Answer from the drawing. Dimensions are ordinates in mm from the lowest x, y and z of the part. Coordinates: 2 decimals unless noted, no trailing zeros. Order: outer loops, then holes, each group sorted by start corner. A loop starts at its lowest first (then second) coordinate and runs counter-clockwise, first axis right, second up. Notation, with made-up numbers: (62, 61) -> (69, 61) arc R28 ccw to (69, 100) -> close; hole circle Ø4 at (39.5, 75). An arc over 180 degrees is marked (long way). Answer in a Markdown table with one row per item.
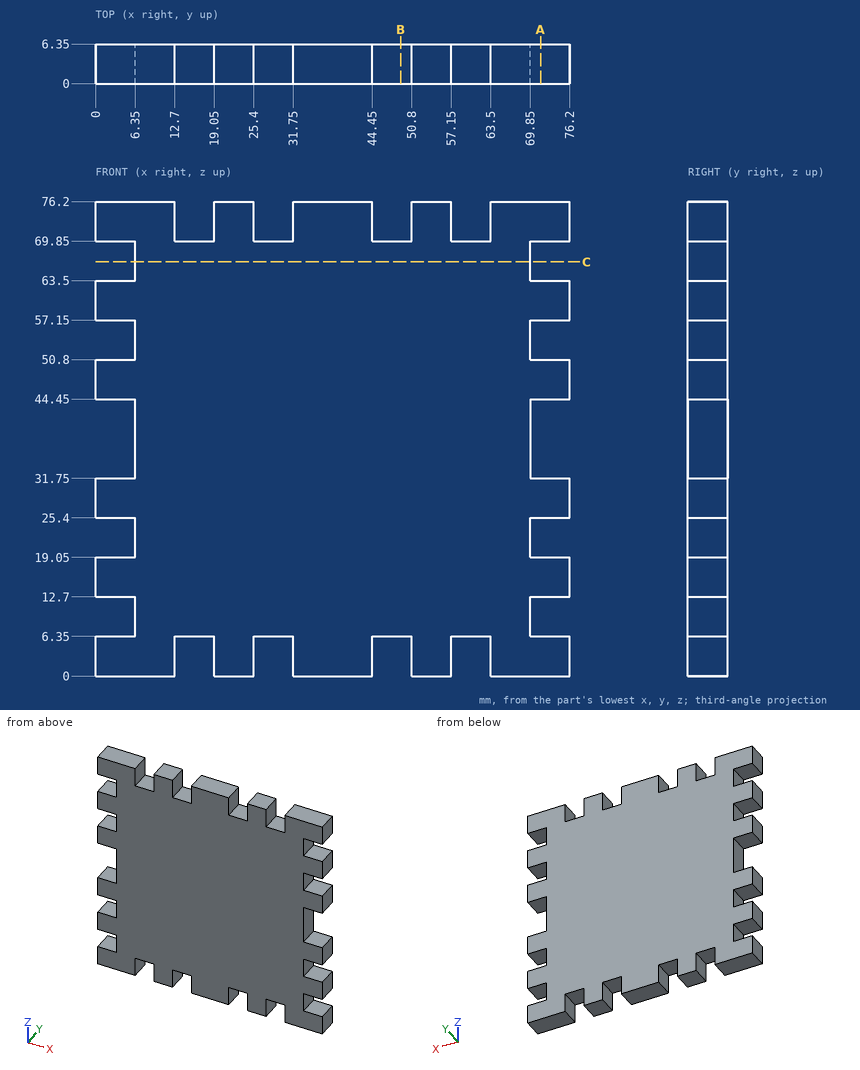
Q1. Consider line 1 (Z direction, x = 71.5, y = 5.25); line 2 (Z direction, x = 18, y = 4). Determine where each line is inside the solid, lowest interval first.
Outcome:
| item | result |
|---|---|
| line 1 | 0 to 6.35, 12.7 to 19.05, 25.4 to 31.75, 44.45 to 50.8, 57.15 to 63.5, 69.85 to 76.2 |
| line 2 | 6.35 to 69.85 |
Q2. The part is cut by section B-B (x = 49). Write down the section's boundary in (y, z).
Outcome:
| item | result |
|---|---|
| outline | (0, 6.35) -> (6.35, 6.35) -> (6.35, 69.85) -> (0, 69.85) -> close |
Q3. The part is cut by section A-A (x = 71.5). Write down the section's boundary in (y, z), then the cut area to 3 significant figures.
Outcome:
| item | result |
|---|---|
| outline | (0, 0) -> (6.35, 0) -> (6.35, 6.35) -> (0, 6.35) -> close; (0, 12.7) -> (6.35, 12.7) -> (6.35, 19.05) -> (0, 19.05) -> close; (0, 25.4) -> (6.35, 25.4) -> (6.35, 31.75) -> (0, 31.75) -> close; (0, 44.45) -> (6.35, 44.45) -> (6.35, 50.8) -> (0, 50.8) -> close; (0, 57.15) -> (6.35, 57.15) -> (6.35, 63.5) -> (0, 63.5) -> close; (0, 69.85) -> (6.35, 69.85) -> (6.35, 76.2) -> (0, 76.2) -> close |
| area | 242 mm² |
Q4. Given pin 1 (3 mm diameter, centred on y = 3, z = 66, fed in from +X); pin 2 (1.9 mm diameter, centred on x = 17.5, y = 3.5, fed in from +Z), each flat-ended and moving along its own axis, determine where each tip first touches the part or whether it passes through.
Outcome:
| item | result |
|---|---|
| pin 1 | x = 69.85 |
| pin 2 | z = 69.85 |
Q5. The part is cut by section C-C (z = 66.5). Write down the section's boundary in (x, y), then the cut area to 3 significant figures.
Outcome:
| item | result |
|---|---|
| outline | (6.35, 0) -> (69.85, 0) -> (69.85, 6.35) -> (6.35, 6.35) -> close |
| area | 403 mm² |
